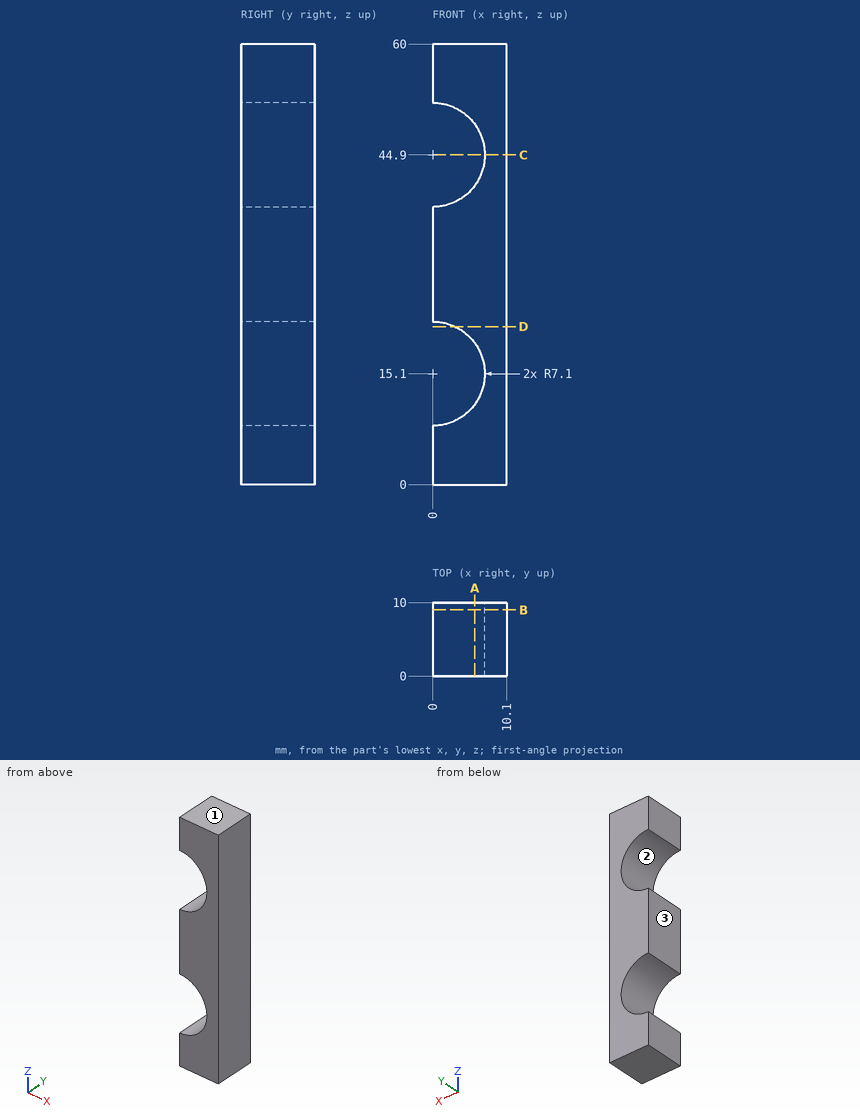
Geometry: see drawing. Coordinates: mm, zero at the bounding-box minimum. Coordinates: 2 decimals unless noted, no trailing zeros. Loops run counter-clockwise (first coordinate to the right, second up) from the corner with the lowest first, then second, coordinate; pieces in that order, holes last. Notation, with made-up numbers: (81.25, 44) -> (85.25, 44) arc R27 cw to (85.25, 76) -> close; hole circle Ø5 at (-17.5, 73). An arc over 180 degrees is marked (long way). Use a Markdown table: item, result.
1) Cut plane C-C (z = 44.9). Return the cut outline in (x, y), then the cut area to 3 significant figures.
Results found:
| item | result |
|---|---|
| outline | (7.1, 0) -> (10.1, 0) -> (10.1, 10) -> (7.1, 10) -> close |
| area | 30.0 mm2 |
2) Cut plane B-B (y = 9). Return the cut outline in (x, z), then the cut area to 3 significant figures.
Results found:
| item | result |
|---|---|
| outline | (0, 0) -> (10.1, 0) -> (10.1, 60) -> (0, 60) -> (0, 52) arc R7.1 cw to (0, 37.8) -> (0, 22.2) arc R7.1 cw to (0, 8) -> close |
| area | 448 mm2 |
3) Cut plane A-A (x = 5.75). Return the cut outline in (y, z), then the cut area to 3 significant figures.
Results found:
| item | result |
|---|---|
| outline | (0, 0) -> (10, 0) -> (10, 10.93) -> (0, 10.93) -> close; (0, 19.27) -> (10, 19.27) -> (10, 40.73) -> (0, 40.73) -> close; (0, 49.07) -> (10, 49.07) -> (10, 60) -> (0, 60) -> close |
| area | 433 mm2 |
4) Contact query for a flat-ended pin moving along its axis: pin 1 (5 mm diameter, centred on x = 3, z = 14, fed in from -Y) (3 decimals). Output: stop coordinate, or through.
Results found:
| item | result |
|---|---|
| pin 1 | passes through |
5) Cut plane D-D (z = 21.5). Return the cut outline in (x, y).
Results found:
| item | result |
|---|---|
| outline | (3.07, 0) -> (10.1, 0) -> (10.1, 10) -> (3.07, 10) -> close |
6) Material intervals for line 1 along Z through (x, y) = (5.25, 3.75); line 2 along Z through (x, y) = (2.25, 5.75); line 3 along X through (y, z) = (4.5, 41.5), sorted ascending. Write a range as from..to.
Results found:
| item | result |
|---|---|
| line 1 | z = 0..10.32, 19.88..40.12, 49.68..60 |
| line 2 | z = 0..8.37, 21.83..38.17, 51.63..60 |
| line 3 | x = 6.23..10.1 |
7) Pull-direction query (Z, two-part tool) for the marked faces 1, 2 and 3; classes: released by +Z, released by -Z, zero draft, split by the parting line, or undercut.
Results found:
| item | result |
|---|---|
| face 1 | released by +Z |
| face 2 | undercut |
| face 3 | zero draft |
